```python
from build123d import *

# Parameters (mm, degrees)
F0_W     = 53.34
F0_H     = 73.66
F0_W_2   = 6.35
F0_H_2   = 12.7
F1_DEPTH = 3.175


with BuildPart() as f1:
    # F0 (on Front) → F1 (new body)
    with BuildSketch(Plane.XZ):
        Polygon((-86.761358, 126.414508), (-91.761358, 126.414508), (-91.761358, -38.685492), (9.838642, -38.685492), (9.838642, 126.414508), (4.838642, 126.414508), (4.838642, 113.714508), (1.638242, 113.714508), (1.638242, 126.414508), (-83.560958, 126.414508), (-83.560958, 113.714508), (-86.761358, 113.714508), align=None)
        with Locations((-41.98038, 29.224732)):
            Rectangle(F0_W, F0_H, mode=Mode.SUBTRACT)
        with Locations((-42.371655, 86.725142)):
            Rectangle(F0_W_2, F0_H_2, mode=Mode.SUBTRACT)
        with Locations((-41.98038, 29.224732)):
            Rectangle(F0_W, F0_H)
    extrude(amount=-F1_DEPTH)


solid = f1.part
```
Verification items for the finished model (mm, model axes). A direction names the side the tool comes from. Coordinates: 2 decimals unless noted, no trailing zeros. Return JSON: item names as keys, results as strings.
1. Tool access check on faces 4 (the flat face through (-45.547, 2, 87)), 5 (the flat face through (-42, 3.175, 45)), 6 (the flat face through (-85, 2, 113.715)). Record the directions out of +Z, -Z, +X, -X, +Y, -Y that give a thin tool (end or side, any length) a straight path to the whole face; none if there is none.
Established:
{"face 4": "+Y, -Y", "face 5": "+Z, -Z, +X, -X, +Y", "face 6": "+Z, +Y, -Y"}
2. Thickness scan on L1, parallel to Z at x = -44, y = 0.3; L2, parallel to X at y = 1.2, z = 84; L3, parallel to Z at x = -85.5, y = 2.45. Record the ranges inside material, lowest first.
Established:
{"L1": "z = -38.69 to 80.38, 93.08 to 126.41", "L2": "x = -91.76 to -45.55, -39.2 to 9.84", "L3": "z = -38.69 to 113.71"}
3. Go/stop test with a flat-tipped pin: pin 1 (1.6 mm diameter, centred on x = 2.5, y = 1.5, fed in from +Z). Record where the tip stops, or that it passes through.
Established:
{"pin 1": "stops at z = 113.71"}
4. Mould release check, pull along X, two halves, no side actions. Record for faces 1 (the flat face through (9.839, 2, 43)), 2 (the flat face through (-89, 2, 126.415)), 3 (the flat face through (-42, 2, 80.375)): +X half, -X half, draft (parallel to the pull), parting line (faces both ways), or undercut.
Established:
{"face 1": "+X half", "face 2": "draft", "face 3": "undercut"}
